For this review, take the finished solid that the model builds, in its own axes (mm). Coordinates: 2 decimals unless noted, no trailing zeros. Write each loop counter-clockwise with the first axis right and the second up, starting at its lowest first coordinate (ties: lowest second). Pieces come first, ordered by that corner, then holes.
Autodesk Inventor part; units mm, degrees
ref_plane "YZ Plane" through (0, 0, 0) normal (1, 0, 0) x (0, 1, 0)
ref_plane "XZ Plane" through (0, 0, 0) normal (0, 1, 0) x (-1, 0, 0)
ref_plane "XY Plane" through (0, 0, 0) normal (0, 0, 1) x (1, 0, 0)
sketch "Sketch1" plane through (0, 0, 0) normal (0, 1, 0) x (-1, 0, 0)
  circle A0 centre (32.6132, 75.9327) radius 1.6
  circle A1 centre (-32.6132, 75.9327) radius 1.6
  circle A2 centre (80.7596, -11.9856) radius 1.6
  circle A3 centre (-80.7596, -11.9856) radius 1.6
  circle A4 centre (80.7596, -11.9856) radius 5
  circle A5 centre (32.6132, 75.9327) radius 5
  circle A6 centre (-32.6132, 75.9327) radius 5
  circle A7 centre (-80.7596, -11.9856) radius 5
  line L0 (-90.2776, 1.5) -> (-46.4378, 77.4327)
  line L1 (46.4378, 77.4327) -> (90.2776, 1.5)
  line L2 (-83.3494, 1.5) -> (-42.9737, 71.4327)
  line L3 (36.6132, 72.9327) -> (40.3756, 72.9327)
  line L4 (42.9737, 71.4327) -> (83.3494, 1.5)
  line L5 (83.3494, -1.5) -> (80.1615, -7.0215)
  line L6 (85.3577, -10.0215) -> (90.2776, -1.5)
  line L7 (43.8397, 78.9327) -> (36.6132, 78.9327)
  line L8 (-17.4338, 72.9327) -> (-28.6132, 72.9327)
  line L9 (-28.6132, 78.9327) -> (28.6132, 78.9327)
  line L10 (-36.6132, 72.9327) -> (-40.3756, 72.9327)
  line L11 (-36.6132, 78.9327) -> (-43.8397, 78.9327)
  line L12 (-83.3494, -1.5) -> (-80.1615, -7.0215)
  line L13 (-85.3577, -10.0215) -> (-90.2776, -1.5)
  line L14 (-80.7596, -11.9856) -> (-77.7596, -11.9856) construction
  line L15 (76.7596, -14.9856) -> (-76.7596, -14.9856)
  arc A8 (90.2776, -1.5) -> (90.2776, 1.5) centre (87.6795, 0) ccw
  arc A9 (83.3494, -1.5) -> (83.3494, 1.5) centre (80.7513, 0) ccw
  arc A10 (46.4378, 77.4327) -> (43.8397, 78.9327) centre (43.8397, 75.9327) ccw
  arc A11 (42.9737, 71.4327) -> (40.3756, 72.9327) centre (40.3756, 69.9327) ccw
  arc A12 (-43.8397, 78.9327) -> (-46.4378, 77.4327) centre (-43.8397, 75.9327) ccw
  arc A13 (-40.3756, 72.9327) -> (-42.9737, 71.4327) centre (-40.3756, 69.9327) ccw
  arc A14 (-83.3494, 1.5) -> (-83.3494, -1.5) centre (-80.7513, 0) ccw
  arc A15 (-90.2776, 1.5) -> (-90.2776, -1.5) centre (-87.6795, 0) ccw
  line L16 (42.9737, 71.4327) -> (45.4737, 67.1025)
  line L17 (45.4737, 67.1025) -> (48.4737, 61.9064)
  line L18 (-42.9737, 71.4327) -> (-45.4737, 67.1025)
  line L19 (-45.4737, 67.1025) -> (-48.4737, 61.9064)
  line L20 (-23.0235, 72.9327) -> (-26.0235, 72.9327)
  line L21 (-23.0235, 72.9327) -> (-20.0235, 72.9327)
  line L22 (-28.0015, 33.4735) -> (-14.8357, 56.2774)
  line L23 (-5.4338, 56.9735) -> (5.4338, 56.9735)
  line L24 (14.8357, 56.2774) -> (28.0015, 33.4735)
  line L25 (5.4338, 6.9735) -> (-5.4338, 6.9735)
  line L26 (-14.8357, 7.6697) -> (-28.0015, 30.4735)
  line L27 (14.4338, 6.1697) -> (14.4338, -5.9856)
  line L28 (-14.4338, 6.1697) -> (-14.4338, -5.9856)
  line L29 (-8.4338, -5.9856) -> (-8.4338, 3.9735)
  line L30 (8.4338, -5.9856) -> (8.4338, 3.9735)
  line L31 (-14.4338, 57.7774) -> (-14.4338, 69.9327)
  line L32 (-8.4338, 69.9327) -> (-8.4338, 59.9735)
  line L33 (14.4338, 57.7774) -> (14.4338, 69.9327)
  line L34 (8.4338, 69.9327) -> (8.4338, 59.9735)
  arc A16 (14.4338, -5.9856) -> (17.4338, -8.9856) centre (17.4338, -5.9856) ccw
  arc A17 (14.8357, 7.6697) -> (14.4338, 6.1697) centre (17.4338, 6.1697) ccw
  arc A18 (8.4338, 3.9735) -> (5.4338, 6.9735) centre (5.4338, 3.9735) ccw
  arc A19 (-5.4338, 6.9735) -> (-8.4338, 3.9735) centre (-5.4338, 3.9735) ccw
  arc A20 (-14.4338, 6.1697) -> (-14.8357, 7.6697) centre (-17.4338, 6.1697) ccw
  arc A21 (-28.0015, 33.4735) -> (-28.0015, 30.4735) centre (-25.4034, 31.9735) ccw
  arc A22 (28.0015, 30.4735) -> (28.0015, 33.4735) centre (25.4034, 31.9735) ccw
  arc A23 (-14.8357, 56.2774) -> (-14.4338, 57.7774) centre (-17.4338, 57.7774) ccw
  arc A24 (-14.4338, 69.9327) -> (-17.4338, 72.9327) centre (-17.4338, 69.9327) ccw
  arc A25 (5.4338, 56.9735) -> (8.4338, 59.9735) centre (5.4338, 59.9735) ccw
  arc A26 (-8.4338, 59.9735) -> (-5.4338, 56.9735) centre (-5.4338, 59.9735) ccw
  arc A27 (14.4338, 57.7774) -> (14.8357, 56.2774) centre (17.4338, 57.7774) ccw
  line L35 (17.4338, 72.9327) -> (28.6132, 72.9327)
  line L36 (5.4338, 72.9327) -> (-5.4338, 72.9327)
  line L37 (5.4338, -8.9856) -> (-5.4338, -8.9856)
  line L38 (-17.4338, -8.9856) -> (-76.7596, -8.9856)
  arc A28 (5.4338, -8.9856) -> (8.4338, -5.9856) centre (5.4338, -5.9856) ccw
  arc A29 (-8.4338, -5.9856) -> (-5.4338, -8.9856) centre (-5.4338, -5.9856) ccw
  arc A30 (-17.4338, -8.9856) -> (-14.4338, -5.9856) centre (-17.4338, -5.9856) ccw
  arc A31 (-5.4338, 72.9327) -> (-8.4338, 69.9327) centre (-5.4338, 69.9327) ccw
  arc A32 (8.4338, 69.9327) -> (5.4338, 72.9327) centre (5.4338, 69.9327) ccw
  arc A33 (17.4338, 72.9327) -> (14.4338, 69.9327) centre (17.4338, 69.9327) ccw
  circle A34 centre (33.4338, 2.3349) radius 6.25
  circle A35 centre (53.4338, 2.3349) radius 6.25
  line L39 (86.5956, -77.4481) -> (86.5956, -51.4481)
  line L40 (86.5956, -51.4481) -> (74.5956, -51.4481)
  line L41 (-25.4034, 31.9735) -> (-28.8675, 31.9735)
  line L42 (-25.4034, 31.9735) -> (-21.9393, 31.9735) construction
  line L43 (-28.8675, 31.9735) -> (-26.3675, 36.3037)
  line L44 (-26.3675, 36.3037) -> (-54.0335, 52.2766)
  arc A36 (63.4338, 16.6554) -> (60.4338, 19.6554) centre (60.4338, 16.6554) ccw
  line L45 (8.4338, -14.9856) -> (23.4338, -14.9856)
  line L46 (63.4338, 16.6554) -> (63.4338, -5.9856)
  line L47 (21.7557, 16.6554) -> (24.2916, 16.6554)
  line L48 (20.4338, 6.1697) -> (20.4338, -5.9856)
  line L49 (20.8357, 7.6697) -> (25.1576, 15.1554)
  line L50 (28.0015, 30.4735) -> (24.3537, 24.1554)
  line L51 (19.1576, 15.1554) -> (14.8357, 7.6697)
  line L52 (17.4338, -8.9856) -> (17.4338, -8.9856)
  line L53 (66.4338, -8.9856) -> (76.7596, -8.9856)
  arc A37 (17.4338, -8.9856) -> (20.4338, -5.9856) centre (17.4338, -5.9856) ccw
  arc A38 (20.8357, 7.6697) -> (20.4338, 6.1697) centre (23.4338, 6.1697) ccw
  arc A39 (25.1576, 15.1554) -> (24.2916, 16.6554) centre (24.2916, 15.6554) ccw
  arc A40 (21.7557, 16.6554) -> (19.1576, 15.1554) centre (21.7557, 13.6554) ccw
  arc A41 (24.3537, 24.1554) -> (26.9518, 19.6554) centre (26.9518, 22.6554) ccw
  arc A42 (63.4338, -5.9856) -> (66.4338, -8.9856) centre (66.4338, -5.9856) ccw
  line L54 (26.9518, 19.6554) -> (60.4338, 19.6554)
  point P0 (0, 0)
  point P1 (0, 0)
  point P2 (45.5718, 78.9327)
  point P3 (91.1436, 0)
  point P4 (0, 0)
  point P5 (-84.2154, 0)
  point P6 (-42.1077, 72.9327)
  point P7 (-76.7596, -8.9856)
  point P8 (-80.8494, -5.8301)
  point P9 (-74.3148, -8.9856)
  point P10 (80.8494, -5.8301)
  point P11 (74.3148, -8.9856)
  point P12 (-63.1615, 36.4663)
  point P13 (-14.4338, 56.9735)
  point P14 (14.4338, 56.9735)
  point P15 (-14.4338, 6.9735)
  point P16 (-14.4338, -8.9856)
  point P17 (-8.4338, -8.9856)
  point P18 (8.4338, -8.9856)
  point P19 (-8.4338, 72.9327)
  point P20 (14.4338, 72.9327)
  point P21 (8.4338, 72.9327)
  point P22 (20.0236, 16.6554)
  point P23 (26.0236, 16.6554)
  dimension "d0" = 3.2
  dimension "d1" = 3.2
  dimension "d2" = 3.2
  dimension "d3" = 10
  dimension "d4" = 10
  dimension "d24" = 3
  dimension "d27" = 5
  dimension "d29" = 6
  dimension "d31" = 5
  dimension "d33" = 6
  dimension "d36" = 3
  dimension "d37" = 3
  dimension "d39" = 50
  dimension "d44" = 3
  dimension "d45" = 26
  dimension "d46" = 12
  dimension "d47" = 180
  dimension "d48" = 5
  dimension "d49" = 90
  dimension "d54" = 6
  dimension "d56" = 3
  dimension "d57" = 1
  dimension "d58" = 3
extrude "Extrusion1" add sketch "Sketch1" along normal blind 3 contours A4 | A4 L5 A9 L4 A11 L3 A5 L7 A10 L1 A8 L6 | L15 A7 L38 A30 L28 A20 L26 A21 L22 A23 L31 A24 L8 A6 L9 A5 L35 A33 L33 A27 L24 A22 L50 A41 L54 A36 L46 A42 L53 A4 | A7 | L13 A15 L0 A12 L11 A6 L10 A13 L2 A14 L12 A7 | A5 | A6
properties part number "Top Plat"
Q1. For probe 1 along Z at (x, y) = (28, 0.75); probe 2 along Z at (x, y) = (4.5, 1.4); probe 3 along X at (y, z) = (0.25, 77), list the stretches that pass through material, from the lowest coordinate up.
Ans:
probe 1: z = -14.99 to -8.99, 30.47 to 33.48, 72.93 to 78.93
probe 2: z = -14.99 to -8.99, 6.97 to 56.97, 72.93 to 78.93
probe 3: x = -46.69 to -33.81, -31.42 to 31.42, 33.81 to 46.69
Q2. Add section D-D (z = 63.5). State the section outline as (x, y) points, then the cut area to 3 significant figures.
Ans:
outline: (-54.48, 0) - (-47.55, 0) - (-47.55, 3) - (-54.48, 3) - close; (-14.43, 0) - (-8.43, 0) - (-8.43, 3) - (-14.43, 3) - close; (8.43, 0) - (14.43, 0) - (14.43, 3) - (8.43, 3) - close; (47.55, 0) - (54.48, 0) - (54.48, 3) - (47.55, 3) - close
area: 77.6 mm2
Q3. Add section A-A (z = 37). State the section outline as (x, y) points, then the cut area to 3 significant figures.
Ans:
outline: (-69.78, 0) - (-62.85, 0) - (-62.85, 3) - (-69.78, 3) - close; (-25.97, 0) - (25.97, 0) - (25.97, 3) - (-25.97, 3) - close; (62.85, 0) - (69.78, 0) - (69.78, 3) - (62.85, 3) - close
area: 197 mm2
Q4. Add section B-B (x = 67.5). State the section outline as (y, z) points.
Ans:
outline: (0, -14.99) - (3, -14.99) - (3, -8.99) - (0, -8.99) - close; (0, 28.95) - (3, 28.95) - (3, 40.95) - (0, 40.95) - close
Q5. Draft analysis for pull direction Z (two halves, no side actions). For faces 1 (the flat face through (-68.05, 1.48, 40)), 2 (the flat face through (1, 3, 22)), 3 (the cylindrical face through (31.087, 1.479, 75.452)), state which applies: +Z half, -Z half, draft (parallel to the pull), parting line (faces both ways), or undercut.
Ans:
face 1: +Z half
face 2: draft
face 3: undercut
Q6. Clearance check with flat-ended pins moving along their axes: pin 1 Ø0.9 at (y, z) = (1.5, -1) entering from -X; pin 2 Ø1.5 at (y, z) = (1, 62) entering from +X; pin 3 Ø0.9 at (x, y) = (-21.5, 1.5) entering from -Z. State where each tip first meets the part, or that it passes through.
Ans:
pin 1: stops at x = -90.63
pin 2: stops at x = 55.78
pin 3: stops at z = -14.99
Q7. Add section C-C (x = 20). State the section outline as (y, z) points, then the cut area to 3 significant figures.
Ans:
outline: (0, -14.99) - (3, -14.99) - (3, -8.99) - (0, -8.99) - close; (0, 16.61) - (3, 16.61) - (3, 47.33) - (0, 47.33) - close; (0, 72.93) - (3, 72.93) - (3, 78.93) - (0, 78.93) - close
area: 128 mm2
